from build123d import *

# Parameters (mm, degrees)
SKETCH1_W                   = 165.1
SKETCH1_H                   = 127
BOSS_EXTRUDE1_DEPTH         = 9.525
SKETCH2_R                   = 19.579444904
CUT_EXTRUDE1_DEPTH          = 209.513154561
BOSS_EXTRUDE3_DEPTH         = 63.5
F_1_2_20_TAPPED_HOLE1_D     = 11.50874
F_1_2_20_TAPPED_HOLE1_DEPTH = 31.75
F_1_2_20_TAPPED_HOLE1_TIP   = 3.45757432


with BuildPart() as part:
    # Sketch1 → Boss-Extrude1 (new body)
    with BuildSketch(Plane(origin=(0, 0, 0), x_dir=(1, 0, 0), z_dir=(0, 1, 0))):
        with Locations((82.55, 63.5)):
            Rectangle(SKETCH1_W, SKETCH1_H)
    extrude(amount=BOSS_EXTRUDE1_DEPTH)

    # Sketch2 → Cut-Extrude1 (cut, through all)
    with BuildSketch(Plane(origin=(0, 9.525, 0), x_dir=(1, 0, 0), z_dir=(0, 1, 0))):
        with Locations(Location((82.55, 63.5, 0), (0, 0, 270))):
            Circle(SKETCH2_R)
    extrude(amount=-CUT_EXTRUDE1_DEPTH, mode=Mode.SUBTRACT)

    # Sketch3 → Boss-Extrude3 (add)
    with BuildSketch(Plane(origin=(0, 9.525, 0), x_dir=(1, 0, 0), z_dir=(0, 1, 0))):
        with BuildLine():
            Line((0, 127), (50.8, 127))
            Line((50.8, 127), (50.8, 101.6))
            ThreePointArc((50.8, 101.6), (43.360512242, 83.639487758), (25.4, 76.2))
            Line((25.4, 76.2), (0, 76.2))
            Line((0, 76.2), (0, 127))
        make_face()
        with BuildLine():
            Line((165.1, 127), (114.3, 127))
            Line((114.3, 127), (114.3, 101.6))
            ThreePointArc((114.3, 101.6), (121.739487758, 83.639487758), (139.7, 76.2))
            Line((139.7, 76.2), (165.1, 76.2))
            Line((165.1, 76.2), (165.1, 127))
        make_face()
    extrude(amount=BOSS_EXTRUDE3_DEPTH)

    # 1/2-20 Tapped Hole1
    with Locations(Plane(origin=(25.4, 73.025, -101.6), x_dir=(0, 0, 1), z_dir=(0, 1, 0))):
        with Locations((0, 0), (0, 114.3)):
            Hole(F_1_2_20_TAPPED_HOLE1_D / 2, depth=F_1_2_20_TAPPED_HOLE1_DEPTH)
            with Locations((0, 0, -(F_1_2_20_TAPPED_HOLE1_DEPTH + F_1_2_20_TAPPED_HOLE1_TIP / 2))):  # 118° drill point
                Cone(0, F_1_2_20_TAPPED_HOLE1_D / 2, F_1_2_20_TAPPED_HOLE1_TIP, mode=Mode.SUBTRACT)


solid = part.part
Here's how the part is built. I have some questions about the finished solid (model axes, mm). A direction names the side the tool comes from. Round coordinates to 2 decimals unless told otherwise and drop trailing zeros. Write each loop counter-clockwise with the first axis right and the second up, starting at its lowest first coordinate (ties: lowest second). Pieces come first, ordered by that corner, then holes. Notation, with made-up numbers: (44.5, 70.25) -> (50.5, 70.25) arc R38 ccw to (50.5, 108.25) -> close; hole circle Ø3 at (82, 21.25). An arc over 180 degrees is marked (long way). One line per item, written item: value.
1) We'd pull the mould along Z, two halves only. Please class faces 6 (the face through (81, 5, 0)), 7 (the face through (138.72, 38.42, -101.82)), 8 (the face through (139, 73.025, -108)): released by +Z, released by -Z, zero draft, split by the parting line, or undercut.
Filled sheet:
face 6: released by +Z
face 7: undercut
face 8: zero draft
2) Suppose I cut it at C-C on x = 82.55. List the corners of the cut face in (y, z) for me (3 decimals).
Filled sheet:
outline: (0, -127) -> (9.525, -127) -> (9.525, -83.079) -> (0, -83.079) -> close; (0, -43.921) -> (9.525, -43.921) -> (9.525, 0) -> (0, 0) -> close
3) If I drill on line 1 (X direction, y = 64, z = -101.6); line 2 (X direction, y = 64, z = -101); line 3 (X direction, y = 21, z = -113.5), over which ranges is the centre line in solid material (lowest first)? Write a range as [from, to].
Filled sheet:
line 1: x = [0, 19.65], [31.15, 50.8], [114.3, 133.95], [145.45, 165.1]
line 2: x = [0, 19.68], [31.12, 50.79], [114.31, 133.98], [145.42, 165.1]
line 3: x = [0, 50.8], [114.3, 165.1]
4) Suppose I cut it at D-D on y = 35.5. List the corners of the cut face in (x, z) for me.
Filled sheet:
outline: (0, -127) -> (50.8, -127) -> (50.8, -101.6) arc R25.4 ccw to (25.4, -76.2) -> (0, -76.2) -> close; (114.3, -127) -> (165.1, -127) -> (165.1, -76.2) -> (139.7, -76.2) arc R25.4 ccw to (114.3, -101.6) -> close
5) Suppose I cut it at A-A on y = 68. List the corners of the cut face in (x, z) for me, plus the area to 3 significant figures.
Filled sheet:
outline: (0, -127) -> (50.8, -127) -> (50.8, -101.6) arc R25.4 ccw to (25.4, -76.2) -> (0, -76.2) -> close; (114.3, -127) -> (165.1, -127) -> (165.1, -76.2) -> (139.7, -76.2) arc R25.4 ccw to (114.3, -101.6) -> close; hole circle Ø11.51 at (25.4, -101.6); hole circle Ø11.51 at (139.7, -101.6)
area: 4,680 mm2
6) I'm going to push a flat-ended pin straight in: pin 1 Ø6 at (x, y) = (27, 24.5) entering from +Z. Where does the tip first touch, or does it pass through?
Filled sheet:
pin 1: stops at z = -76.2
7) For faces 1 (the face through (0, 36, -91)), 2 (the face through (121.54, 40.83, -83.84)), 3 (the face through (145.405, 56.928, -100.851)), 4 (the face through (152, 41, -76.2)), 5 (the face through (50.8, 41, -114)), which set-ups out of +Z, -Z, +X, -X, +Y, -Y let a thin tool reach every point of the face, with its end or its side?
Filled sheet:
face 1: +Z, -Z, -X, +Y, -Y
face 2: +Z, +Y
face 3: +Y
face 4: +Z, +X, -X, +Y
face 5: +Z, -Z, +Y
8) Suppose I cut it at B-B on z = -63.5. List the corners of the cut face in (x, y) for me (3 decimals), plus the area to 3 significant figures.
Filled sheet:
outline: (0, 0) -> (62.971, 0) -> (62.971, 9.525) -> (0, 9.525) -> close; (102.129, 0) -> (165.1, 0) -> (165.1, 9.525) -> (102.129, 9.525) -> close
area: 1,200 mm2
